```python
from build123d import *

# Parameters (mm, degrees)
CROQUIS1_W              = 75
CROQUIS1_H              = 50
SALIENTE_EXTRUIR1_DEPTH = 42
CROQUIS2_R              = 5.939733441
SALIENTE_EXTRUIR2_DEPTH = 16


with BuildPart() as part:
    # Croquis1 → Saliente-Extruir1 (new body)
    with BuildSketch(Plane.XY):
        Rectangle(CROQUIS1_W, CROQUIS1_H)
    extrude(amount=-SALIENTE_EXTRUIR1_DEPTH)

    # Croquis2 → Saliente-Extruir2 (add)
    with BuildSketch(Plane.XY):
        with Locations(Location((18.830639627, 12, 0), (0, 0, 180))):
            Circle(CROQUIS2_R)
    extrude(amount=SALIENTE_EXTRUIR2_DEPTH)


solid = part.part
```
Geometry check sheet. Reference: the model listing, model coordinates, mm. A direction names the side the tool comes from. Give positions to 0.01 mm unless a question says otherwise; leave off trailing zeros. Order: outer loops, then holes, each group sorted by start corner. A loop starts at its lowest first (then second) coordinate and runs counter-clockwise, first axis right, second up.
1. Section check A-A, the plane y = 12. Enter the section's corners in (x, z).
2. Thickness scan on L1, parallel to Z at x = -10.5, y = -12. Record the ranges inside material, lowest first.
3. Section check C-C, the plane y = -14. Enter the section's corners in (x, z).
4. Section check B-B, the plane x = 22.5. Enter the section's corners in (y, z), and give its area (3 significant figures).
5. Gauge pin test, flat ends, axial feed: pin 1 Ø10 at (x, z) = (-18, 8.5) entering from -Y; pin 2 Ø5 at (x, y) = (24.5, -7) entering from +Z. Record the tip position at first contact, or that the pin passes through.
6. Access from +Z, -Z, +X, -X, +Y, -Y to the whole of each face (thin tool, end or side, straight path). Record for faces 1 (the face through (-1, 25, -21)), 2 (the face through (24.765, 11.739, 7.888)).
Values follow:
1. outline: (-37.5, -42) - (37.5, -42) - (37.5, 0) - (24.77, 0) - (24.77, 16) - (12.89, 16) - (12.89, 0) - (-37.5, 0) - close
2. L1: z = -42 to 0
3. outline: (-37.5, -42) - (37.5, -42) - (37.5, 0) - (-37.5, 0) - close
4. outline: (-25, -42) - (25, -42) - (25, 0) - (16.67, 0) - (16.67, 16) - (7.33, 16) - (7.33, 0) - (-25, 0) - close
4. area: 2,250 mm2
5. pin 1: passes through
5. pin 2: stops at z = 0
6. face 1: +Z, -Z, +X, -X, +Y
6. face 2: +Z
